Can you work these out from the drawing? Everything is in mm from the part's minimum corner. Round coordinates to 2 decimals unless told otherwise and drop trailing zeros. Order: outer loops, then holes, each group sorted by start corner. A loop starts at its lowest first (then second) coordinate and runs counter-clockwise, first axis right, second up. Notation, with made-up numbers: (-37, -0.5) - (-21, -0.5) arc R25 ccw to (-21, 30.5) - close; hole circle Ø4 at (-38, 35). An arc over 180 degrees is marked (long way). Answer as a JSON object with one key per item and string values.
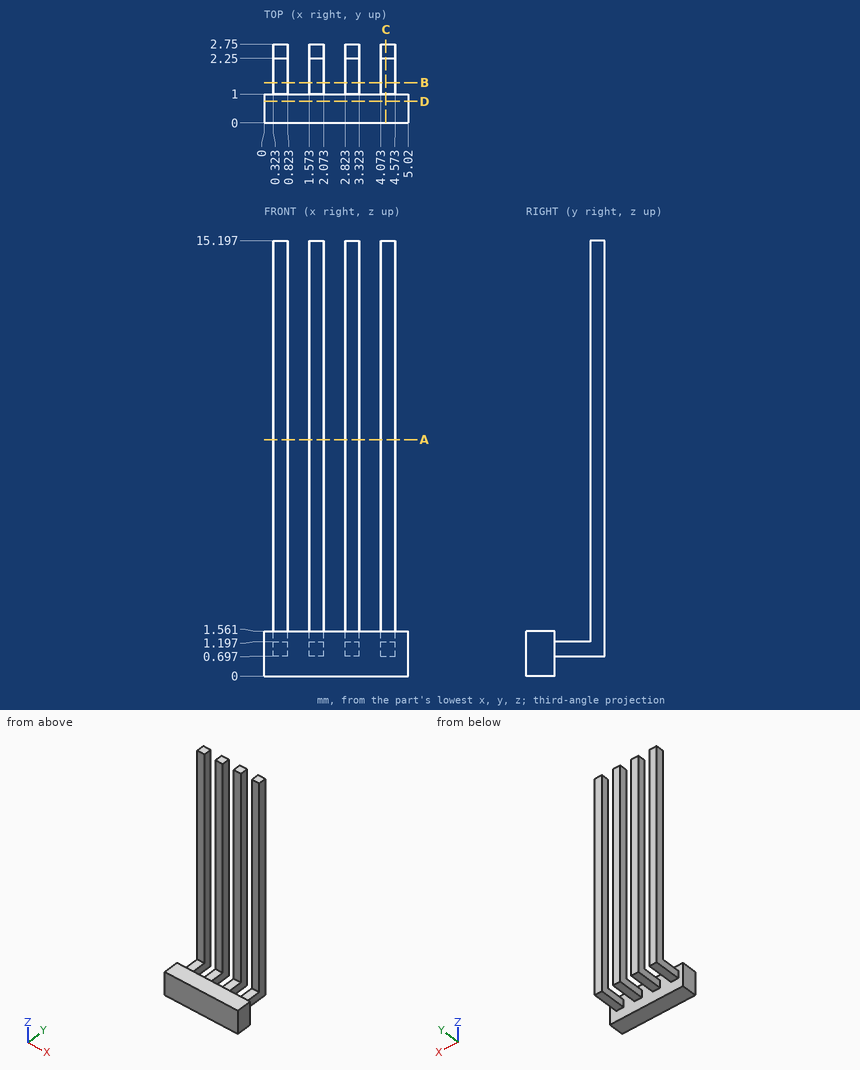
1. Imagine slicing it at D-D (y = 0.75). List the corners of the cut face in (x, z) for me.
Responses:
{"outline": "(0, 0) - (5.02, 0) - (5.02, 1.56) - (0, 1.56) - close"}
2. If I drill on L1, parallel to Y at x = 4.4, z = 11.25; L2, parallel to Z at x = 3.4, y = 0.1; L3, parallel to Z at x = 0.45, y = 1.5, over which ranges is the centre line in solid material (lowest first)? Write a range as [from, to].
Responses:
{"L1": "[2.25, 2.75]", "L2": "[0, 1.56]", "L3": "[0.7, 1.2]"}
3. Imagine slicing it at A-A (z = 8.25). List the corners of the cut face in (x, y) for me.
Responses:
{"outline": "(0.32, 2.25) - (0.82, 2.25) - (0.82, 2.75) - (0.32, 2.75) - close; (1.57, 2.25) - (2.07, 2.25) - (2.07, 2.75) - (1.57, 2.75) - close; (2.82, 2.25) - (3.32, 2.25) - (3.32, 2.75) - (2.82, 2.75) - close; (4.07, 2.25) - (4.57, 2.25) - (4.57, 2.75) - (4.07, 2.75) - close"}
4. Imagine slicing it at B-B (y = 1.4). List the corners of the cut face in (x, z) for me.
Responses:
{"outline": "(0.32, 0.7) - (0.82, 0.7) - (0.82, 1.2) - (0.32, 1.2) - close; (1.57, 0.7) - (2.07, 0.7) - (2.07, 1.2) - (1.57, 1.2) - close; (2.82, 0.7) - (3.32, 0.7) - (3.32, 1.2) - (2.82, 1.2) - close; (4.07, 0.7) - (4.57, 0.7) - (4.57, 1.2) - (4.07, 1.2) - close"}
5. For P1, Ø2, axis at x = 3.5, z = 3.5, coming from the -Y side; P2, Ø1.4, axis at y = 2, z = 7, coming from the -X side; P3, Ø1.4, axis at y = 2, z = 11.5, coming from the +X side, each with a flat end and sliding along its axis, tell me the tip position at first contact or that it passes through.
Responses:
{"P1": "y = 2.25", "P2": "x = 0.32", "P3": "x = 4.57"}
6. Imagine slicing it at C-C (x = 4.25). List the corners of the cut face in (y, z) for me.
Responses:
{"outline": "(0, 0) - (1, 0) - (1, 0.7) - (2.75, 0.7) - (2.75, 15.2) - (2.25, 15.2) - (2.25, 1.2) - (1, 1.2) - (1, 1.56) - (0, 1.56) - close"}
